Autodesk Inventor part; units mm, degrees
ref_plane "YZ Plane" through (0, 0, 0) normal (1, 0, 0) x (0, 1, 0)
ref_plane "XZ Plane" through (0, 0, 0) normal (0, 1, 0) x (-1, 0, 0)
ref_plane "XY Plane" through (0, 0, 0) normal (0, 0, 1) x (1, 0, 0)
sketch "Sketch1" plane through (0, 0, 0) normal (0, 1, 0) x (-1, 0, 0)
  line L0 (0, 0) -> (30, 0)
  line L1 (30, 0) -> (30, -50)
  line L2 (30, -50) -> (0, -50)
  line L3 (0, -50) -> (0, 0)
  dimension "d0" = 30
  dimension "d1" = 50
extrude "Extrusion1" add sketch "Sketch1" along normal blind 5.65
sketch "Sketch2" plane through (-30, 0, 0) normal (0, 0, 1) x (1, 0, 0)
  line L0 (30, 0) -> (0, 0)
  line L1 (30, 0) -> (30, 5.65)
  line L2 (0, 5.65) -> (30, 5.65)
  line L3 (0, 0) -> (0, 5.65)
  line L4 (30, 0) -> (0, 0)
  line L5 (30, 0) -> (27, 0)
  line L6 (27, 0) -> (27, 1.5)
  line L7 (27, 1.5) -> (30, 1.5)
  line L8 (30, 1.5) -> (30, 0)
  line L9 (30, 5.65) -> (27, 5.65)
  line L10 (27, 5.65) -> (27, 4.15)
  line L11 (27, 4.15) -> (30, 4.15)
  line L12 (30, 4.15) -> (30, 5.65)
  dimension "d4" = 3
  dimension "d5" = 1.5
  dimension "d6" = 3
  dimension "d7" = 1.5
extrude "Extrusion2" cut sketch "Sketch2" against normal up to surface (50 mm away) contours L0 L6 L7 L1 | L11 L10 L2 L1
move faces "Move1" translate (0, -0.1, 0) faces at (-2, 4.15, -16.6667)
move faces "Move2" translate (0, 0.1, 0) faces at (-1, 1.5, -16.6667)
properties part number "Maze Wall Middle"
The model under review builds one solid part; all positions refer to its coordinate system, in mm. A direction names the side the tool comes from. Coordinates: 2 decimals unless noted, no trailing zeros. Write each loop counter-clockwise with the first axis right and the second up, starting at its lowest first coordinate (ties: lowest second). Pieces come first, ordered by that corner, then holes. Notation, with made-up numbers: (69.25, 31.5) - (101.25, 31.5) arc R12 cw to (101.25, 39.5) - close; hole circle Ø4 at (11.25, 45.25). An arc over 180 degrees is marked (long way). Answer as a JSON object with one key per item and string values. Group by question number.
1. Add section B-B (y = 0.6). Give the boundary of the cut face in (x, z), plus the area to 3 significant figures.
2. Clearance check with flat-ended pins moving along their axes: pin 1 Ø0.5 at (y, z) = (1, -27.5) entering from +X; pin 2 Ø0.9 at (x, z) = (-1, -29) entering from -Y; pin 3 Ø1.5 at (x, z) = (-1.5, -35.5) entering from +Y. State where each tip first meets the part, or that it passes through.
3. To check wall thickness, follow probe 1 along X at (y, z) = (0.5, -10). State the ranges of the line that lie inside material, in increasing order.
4. Add section A-A (z = -46). Give the boundary of the cut face in (x, y), plus the area to 3 significant figures.
5. Machinability: for faces 1 (the face through (-2, 1.6, -25)), 2 (the face through (0, 3, -25)), 3 (the face through (-2, 4.05, -25)), which of the approach directions +Z, -Z, +X, -X, +Y, -Y give a long, thin tool a straight path to every point of the face, cutting with its end or side? Answer none if there is none.
Findings:
{
 "1": {"outline": "(-30, -50) - (-3, -50) - (-3, 0) - (-30, 0) - close", "area": "1,350 mm²"},
 "2": {"pin 1": "x = -3", "pin 2": "y = 1.6", "pin 3": "y = 4.05"},
 "3": {"probe 1": "-30 to -3"},
 "4": {"outline": "(-30, 0) - (-3, 0) - (-3, 1.6) - (0, 1.6) - (0, 4.05) - (-3, 4.05) - (-3, 5.65) - (-30, 5.65) - close", "area": "160 mm²"},
 "5": {"face 1": "+Z, -Z, +X, -Y", "face 2": "+Z, -Z, +X, +Y, -Y", "face 3": "+Z, -Z, +X, +Y"}
}
